Part model, mm, in its own coordinate system. A direction names the side the tool comes from. Coordinates: 2 decimals unless noted, no trailing zeros. Write each loop counter-clockwise with the first axis right and the second up, starting at its lowest first coordinate (ties: lowest second). Pieces come first, ordered by that corner, then holes. Notation, with made-up numbers: (-13.5, 57) - (18.5, 57) arc R21 ccw to (18.5, 68) - close; hole circle Ø11 at (-31.5, -17). An arc over 180 degrees is marked (long way). Write each question's results on one line, items separated by ' | '.
Autodesk Inventor part; units mm, degrees
ref_plane "YZ Plane" through (0, 0, 0) normal (1, 0, 0) x (0, 1, 0)
ref_plane "XZ Plane" through (0, 0, 0) normal (0, 1, 0) x (-1, 0, 0)
ref_plane "XY Plane" through (0, 0, 0) normal (0, 0, 1) x (1, 0, 0)
sketch "Sketch1" plane through (0, 0, 0) normal (0, 1, 0) x (-1, 0, 0)
  line L0 (-6, 11.25) -> (-6, -11.25)
  line L1 (-6, -11.25) -> (6, -11.25)
  line L2 (6, -11.25) -> (6, 11.25)
  line L3 (6, 11.25) -> (-6, 11.25)
  line L4 (-6, 11.25) -> (6, -11.25) construction
  line L5 (-6, -11.25) -> (6, 11.25) construction
  line L6 (-6, 16) -> (-6, -16)
  line L7 (-6, -16) -> (6, -16)
  line L8 (6, -16) -> (6, 16)
  line L9 (6, 16) -> (-6, 16)
  line L10 (-6, 16) -> (6, -16) construction
  line L11 (-6, -16) -> (6, 16) construction
  circle A0 centre (0, -5.25) radius 6
  circle A1 centre (0, -5.25) radius 2.5
  circle A2 centre (0, 0.75) radius 2.75
  line L12 (0, 16) -> (0, 14)
  circle A3 centre (0, 14) radius 1
  line L13 (0, -16) -> (0, -14)
  circle A4 centre (0, -14) radius 1
  point P0 (0, 0)
  point P1 (-2.6768, 0.1198)
  point P2 (2.6768, 0.1198)
  dimension "d11" = 22.5
  dimension "d12" = 12
  dimension "d13" = 32
  dimension "d18" = 6
  dimension "d19" = 5
  dimension "d20" = 5.5
  dimension "d25" = 2
  dimension "d26" = 2
  dimension "d27" = 2
  dimension "d28" = 2
extrude "Extrusion1" add sketch "Sketch1" along normal blind 4 and the other way blind 18 contours L3 L2 A0 A2 L0 | A0 L1 L0 | A0 A2 | A2 A0 | A0 A2 | A0 L2 L1 | A1
extrude "Extrusion3" add sketch "Sketch1" along normal blind 2.5 contours L3 L2 A0 A2 L0 | L6 L9 L8 L3 | A0 L1 L0 | A0 A2 | L1 L8 L7 L6 | A2 A0 | A0 A2 | A0 L2 L1 | A1
extrude "Extrusion4" add sketch "Sketch1" along normal blind 9.5 contours A0 A2 | A2 A0 | A0 A2 | A1
extrude "Extrusion5" add sketch "Sketch1" along normal blind 13.5 contours A1
sketch "Sketch3" plane through (-6, -18, -11.25) normal (-1, 0, 0) x (0, 0, 1)
  line L0 (0, 0) -> (0, 18)
  line L1 (0, 0) -> (0, 18)
  line L2 (-4.75, 20.5) -> (0, 20.5)
  line L3 (0, 18) -> (0, 20.5)
  line L4 (0, 22) -> (6, 22)
  line L5 (0, 20.5) -> (0, 22)
  line L6 (-3.75, 20.5) -> (-3.75, 18)
  line L7 (-3.75, 20.5) -> (-1.75, 20.5)
  line L8 (-1.75, 20.5) -> (-1.75, 18)
  line L9 (22.5, 0) -> (0, 0)
  line L10 (0, 0) -> (22.5, 0)
  point P0 (11.25, 18)
  dimension "d29" = 2.5
  dimension "d31" = 18
  dimension "d32" = 1.5
  dimension "d33" = 4.75
  dimension "d34" = 2
  dimension "d35" = 1
  dimension "d36" = 22.5
sketch "Sketch4" plane through (6, -18, -11.25) normal (0, 0, -1) x (-1, 0, 0)
  line L0 (0, 0) -> (12, 0)
  line L1 (0, 0) -> (3.8, 0)
  line L2 (3.8, 0) -> (3.8, 3.5)
  line L3 (3.8, 3.5) -> (3.8, 5.5)
  line L4 (3.8, 5.5) -> (8.2, 5.5)
  line L5 (8.2, 5.5) -> (8.2, 3.5)
  line L6 (8.2, 3.5) -> (3.8, 3.5)
  point P0 (6, 18)
  dimension "d37" = 3.8
  dimension "d38" = 3.5
  dimension "d39" = 2
  dimension "d40" = 4.4
extrude "Extrusion6" add sketch "Sketch4" along normal blind 5
properties part number "servo" material "Acetal Resin, Black"
(1) Wall check: line 1 (Z direction, x = 0, y = 1.95); line 2 (Y direction, x = -4.5, z = -3); line 3 (Y direction, x = -5, z = 4). Give the ranges that are in metal, low to high. Write a range as from..to.
Return value:
line 1: z = -16..-15, -13..13, 15..16 | line 2: y = -18..9.5 | line 3: y = -18..4
(2) Two-plate mould, pull along Y, no slides. Class faces 6 (the flat face through (0, -13, -16.25)), 7 (the flat face through (0.1, 0, -12.5)), 8 (the flat face through (0, -9, -11.25)), 9 (the flat face through (0.1, 2.5, -12.5)): released by +Y, released by -Y, zero draft, split by the parting line, or undercut.
Return value:
face 6: zero draft | face 7: undercut | face 8: undercut | face 9: released by +Y
(3) Saw through at B-B on y = -14. Write the cut outline in (x, z).
Return value:
outline: (-6, -11.25) - (-2.2, -11.25) - (-2.2, -16.25) - (2.2, -16.25) - (2.2, -11.25) - (6, -11.25) - (6, 11.25) - (-6, 11.25) - close
(4) Saw through at C-C on z = 13.5. Write the cut outline in (x, y).
Return value:
outline: (-6, 0) - (-0.87, 0) - (-0.87, 2.5) - (-6, 2.5) - close; (0.87, 0) - (6, 0) - (6, 2.5) - (0.87, 2.5) - close
(5) Saw through at A-A on z = -14. Write the cut outline in (x, y).
Return value:
outline: (-6, 0) - (-1, 0) - (-1, 2.5) - (-6, 2.5) - close; (-2.2, -14.5) - (2.2, -14.5) - (2.2, -12.5) - (-2.2, -12.5) - close; (1, 0) - (6, 0) - (6, 2.5) - (1, 2.5) - close
(6) Flat gauge pins, fed straight in: P1, Ø3, axis at x = -3.5, z = 8, coming from the +Y side; P2, Ø6, axis at x = -2.5, z = 3, coming from the +Y side; P3, Ø3, axis at x = 0, z = 14, coming from the -Y side; P4, Ø5, axis at x = -4, z = -7.5, coming from the +Y side. Where does each tip first touch, or does it go through?
Return value:
P1: stops at y = 4 | P2: stops at y = 9.5 | P3: stops at y = 0 | P4: stops at y = 13.5
(7) Saw through at D-D on z = 0.75. Write the cut outline in (x, y).
Return value:
outline: (-6, -18) - (6, -18) - (6, 4) - (2.75, 4) - (2.75, 9.5) - (-2.75, 9.5) - (-2.75, 4) - (-6, 4) - close
(8) 3-axis set-ups, long thin cutter, end or side, ignore diameter. For faces 1 (the flat face through (0, 3, 11.25)), 2 (the flat face through (5, 4, -10)), 3 (the flat face through (0, -12.5, -14)), 4 (the flat face through (-5, 4, -10)), 5 (the flat face through (0, 9.5, -2)): which of +Z, -Z, +X, -X, +Y, -Y reach the whole face in a straight line?
Return value:
face 1: +Z, +X, -X, +Y | face 2: -Z, +X, +Y | face 3: -Z, +X, -X | face 4: -Z, -X, +Y | face 5: +Y
